Geometry check sheet. Reference: the model listing, model coordinates, mm. A direction names the side the tool comes from. Give positions to 0.01 mm unless a question says otherwise; leave off trailing zeros. Order: outer loops, then holes, each group sorted by start corner. A loop starts at its lowest first (then second) coordinate and runs counter-clockwise, first axis right, second up. Notation, with made-up numbers: (37, -28) - (94, -28) arc R22 cw to (94, -5) - close; hole circle Ø5 at (-21, -3.5). An arc over 180 degrees is marked (long way). Put each result on its own line as item: value. Start each with the question number.
```python
from build123d import *

# Parameters (mm, degrees)
CROQUIS1_W              = 102
CROQUIS1_H              = 58
SALIENTE_EXTRUIR1_DEPTH = 2
CROQUIS2_W              = 91
CROQUIS2_H              = 46
SALIENTE_EXTRUIR2_DEPTH = 3
CROQUIS3_W              = 90
CROQUIS3_H              = 50
SALIENTE_EXTRUIR3_DEPTH = 20
CROQUIS4_R              = 1.85
CORTAR_EXTRUIR1_DEPTH   = 62.983868869


with BuildPart() as part:
    # Croquis1 → Saliente-Extruir1 (new body)
    with BuildSketch(Plane(origin=(0, 0, 0), x_dir=(1, 0, 0), z_dir=(0, 1, 0))):
        Rectangle(CROQUIS1_W, CROQUIS1_H)
    extrude(amount=SALIENTE_EXTRUIR1_DEPTH)

    # Croquis2 → Saliente-Extruir2 (add)
    with BuildSketch(Plane(origin=(0, 2, 0), x_dir=(1, 0, 0), z_dir=(0, 1, 0))):
        Rectangle(CROQUIS2_W, CROQUIS2_H)
    extrude(amount=SALIENTE_EXTRUIR2_DEPTH)

    # Croquis3 → Saliente-Extruir3 (add)
    with BuildSketch(Plane.XZ):
        Rectangle(CROQUIS3_W, CROQUIS3_H)
    extrude(amount=SALIENTE_EXTRUIR3_DEPTH)

    # Croquis4 → Cortar-Extruir1 (cut, through all)
    with BuildSketch(Plane.XZ):
        with Locations(Location((-45, 24, 0), (0, 0, 270))):
            Circle(CROQUIS4_R)
        with Locations(Location((45, 24, 0), (0, 0, 270))):
            Circle(CROQUIS4_R)
        with Locations(Location((-48, -26, 0), (0, 0, 270))):
            Circle(CROQUIS4_R)
        with Locations(Location((48, -26, 0), (0, 0, 270))):
            Circle(CROQUIS4_R)
    extrude(amount=-CORTAR_EXTRUIR1_DEPTH, mode=Mode.SUBTRACT)


solid = part.part
```
Item 1: Cross-section at D-D (x = -38). Enter the section's corners in (y, z).
Item 2: Thickness scan on line 1 along X through (y, z) = (1.15, 24); line 2 along Z through (x, y) = (45, 1.5); line 3 along X through (y, z) = (-2, -3.5). Record the ranges inside material, lowest first.
Item 3: Cross-section at C-C (z = 24). Enter the section's corners in (x, y), and give its area (3 significant figures).
Item 4: Release check for a two-part mould opening along Z. For faces 6 (the face through (-44, 0, 24)), 7 (the face through (-1, -10, 25)), 8 (the face through (-44.444, 1.354, 22.235)), 9 (the face through (-45, -10, 0)) record: +Z half, -Z half, draft (parallel to the pull), parting line (faces both ways), or undercut.
Item 5: Cross-section at A-A (z = -26). Enter the section's corners in (x, y).
Item 6: Gauge pin test, flat ends, axial feed: pin 1 Ø1.5 at (x, y) = (-26, -11.5) entering from -Z; pin 2 Ø6 at (x, z) = (48, -26) entering from +Y; pin 3 Ø3 at (y, z) = (-11.5, 3) entering from -X. Record the tip position at first contact, or that the pin passes through.
Item 7: Set-up check for faces 1 (the face through (-45.5, 3, 0)), 2 (the face through (44.29, 1.35, 22.29)), 3 (the face through (-1, 3, -23)), 4 (the face through (-1, -10, -25)), 5 (the face through (-1, 3, 23)): record each of +Z, -Z, +X, -X, +Y, -Y from which the full face is reachable in a straight line by a thin tool's end or side.
Item 8: Cross-section at B-B (x = 48). Enter the section's corners in (y, z).
Recorded:
1. outline: (-20, -25) - (0, -25) - (0, -29) - (2, -29) - (2, -23) - (5, -23) - (5, 23) - (2, 23) - (2, 29) - (0, 29) - (0, 25) - (-20, 25) - close
2. line 1: x = -51 to -46.85, -43.15 to 43.15, 46.85 to 51
2. line 2: z = -29 to 22.15, 25.85 to 29
2. line 3: x = -45 to 45
3. outline: (-51, 0) - (-46.85, 0) - (-46.85, 2) - (-51, 2) - close; (-45, -20) - (45, -20) - (45, 0) - (43.15, 0) - (43.15, 2) - (-43.15, 2) - (-43.15, 0) - (-45, 0) - close; (46.85, 0) - (51, 0) - (51, 2) - (46.85, 2) - close
3. area: 1,990 mm^2
4. face 6: undercut
4. face 7: +Z half
4. face 8: undercut
4. face 9: draft
5. outline: (-51, 0) - (-49.85, 0) - (-49.85, 2) - (-51, 2) - close; (-46.15, 0) - (46.15, 0) - (46.15, 2) - (-46.15, 2) - close; (49.85, 0) - (51, 0) - (51, 2) - (49.85, 2) - close
6. pin 1: stops at z = -25
6. pin 2: stops at y = 2
6. pin 3: stops at x = -45
7. face 1: +Z, -Z, -X, +Y
7. face 2: +Y
7. face 3: -Z, +X, -X, +Y
7. face 4: -Z, +X, -X, -Y
7. face 5: +Z, +X, -X, +Y
8. outline: (0, -29) - (2, -29) - (2, -27.85) - (0, -27.85) - close; (0, -24.15) - (2, -24.15) - (2, 29) - (0, 29) - close
